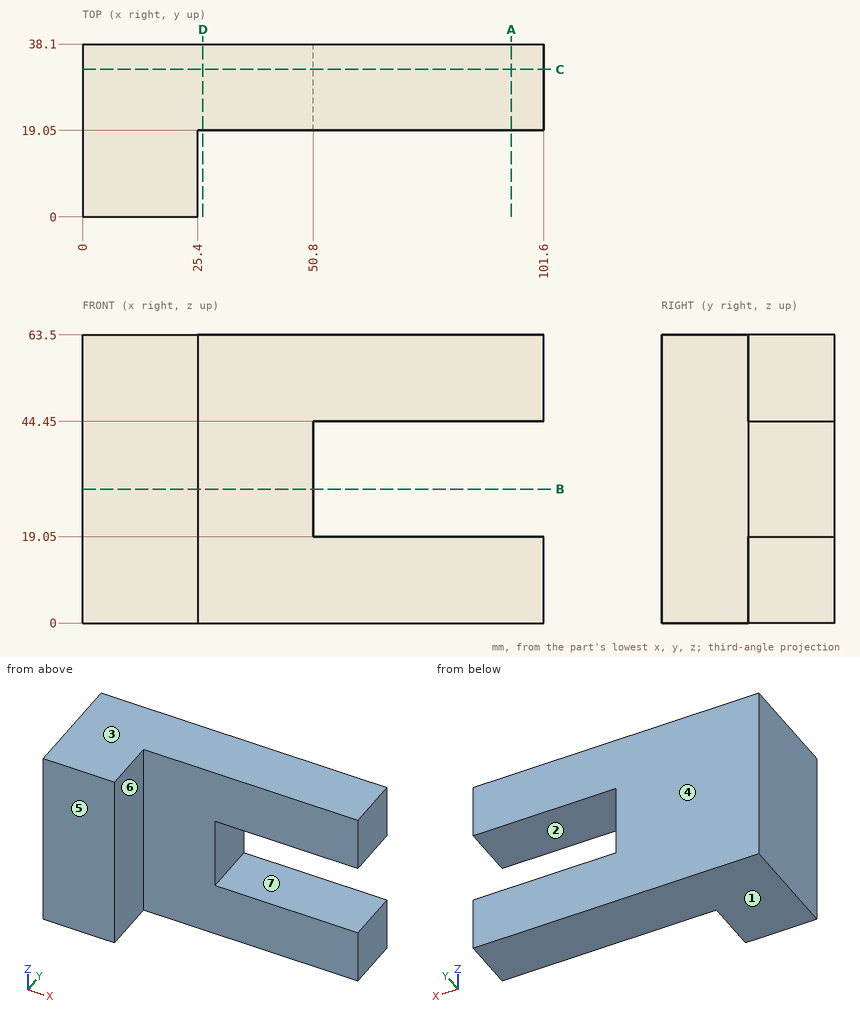
Design review of the part shown in the three views and the two pictorial views. Dimensions are in mm from the part's minimum x, y and z. A direction names the side the tool comes from. Round coordinates to 2 decimals unless told otherwise and drop trailing zeros. Loops run counter-clockwise (first coordinate to the right, second up) from the corner with the lowest first, then second, coordinate; pieces in that order, holes last. Notation, with made-up numbers: (61, 5.5) - (106, 5.5) arc R13 ccw to (106, 26.5) - close; hole circle Ø11 at (24.25, -31.5). An arc over 180 degrees is marked (long way). Answer as CSV lines item,"result".
(1) Consider section D-D on x = 26.5. Give the boundary of the cut face in (y, z), then the cut area to 3 significant figures.
Checked values:
outline,"(19.05, 0) - (38.1, 0) - (38.1, 63.5) - (19.05, 63.5) - close"
area,"1,210 mm2"
(2) Wall thickness on line 1 (Z direction, x = 62.5, y = 35); line 2 (Y direction, x = 82, z = 53.5); line 3 (X direction, y = 29, z = 28): over which ranges is each line inside the solid? List them lowest first.
Checked values:
line 1,"z = 0 to 19.05, 44.45 to 63.5"
line 2,"y = 19.05 to 38.1"
line 3,"x = 0 to 50.8"
(3) Mouldability with a two-part tool opening along Z and no side actions: class the marked faces 1, 2, 3 and 4 as +Z half, -Z half, draft (parallel to the pull), parting line (faces both ways), or undercut.
Checked values:
face 1,"-Z half"
face 2,"undercut"
face 3,"+Z half"
face 4,"draft"
(4) Tool access review of the marked faces 5, 6 and 7: name each direction out of +Z, -Z, +X, -X, +Y, -Y from which nothing blocks a thin tool from reaching the whole face with its end or side.
Checked values:
face 5,"+Z, -Z, +X, -X, -Y"
face 6,"+Z, -Z, +X, -Y"
face 7,"+X, +Y, -Y"
(5) Consider section A-A on x = 94.5. Give the boundary of the cut face in (y, z), then the cut area to 3 significant figures.
Checked values:
outline,"(19.05, 0) - (38.1, 0) - (38.1, 19.05) - (19.05, 19.05) - close; (19.05, 44.45) - (38.1, 44.45) - (38.1, 63.5) - (19.05, 63.5) - close"
area,"726 mm2"
(6) Consider section B-B on z = 29.5. Give the boundary of the cut face in (x, y), then the cut area to 3 significant figures.
Checked values:
outline,"(0, 0) - (25.4, 0) - (25.4, 19.05) - (50.8, 19.05) - (50.8, 38.1) - (0, 38.1) - close"
area,"1,450 mm2"
(7) Insertion check: P1, Ø19, axis at x = 51, z = 36, coming from the -Y side; P2, Ø5, axis at y = 17, z = 30, coming from the +X side; P3, Ø3, axis at y = 14, z = 48.5, coming from the +X side. Each pin has a flat end and moves straight along its axis. Give the tip position at first contact, or say it passes through.
Checked values:
P1,"stops at y = 19.05"
P2,"stops at x = 50.8"
P3,"stops at x = 25.4"
(8) Consider section C-C on y = 32.5. Give the boundary of the cut face in (x, z), then the cut area to 3 significant figures.
Checked values:
outline,"(0, 0) - (101.6, 0) - (101.6, 19.05) - (50.8, 19.05) - (50.8, 44.45) - (101.6, 44.45) - (101.6, 63.5) - (0, 63.5) - close"
area,"5,160 mm2"
